from build123d import *

# Parameters (mm, degrees)
SKETCH9_R           = 25
BOSS_EXTRUDE7_DEPTH = 10


with BuildPart() as part:
    # Sketch9 → Boss-Extrude7 (new, symmetric)
    with BuildSketch(Plane(origin=(0, 0, 0), x_dir=(1, 0, 0), z_dir=(0, 1, 0))):
        with BuildLine():
            Line((0, -240), (140, -240))
            Line((140, -240), (43.894055239, 23.943932732))
            ThreePointArc((43.894055239, 23.943932732), (0, 50), (-43.894055239, 23.943932732))
            Line((-43.894055239, 23.943932732), (-140, -240))
            Line((-140, -240), (0, -240))
        make_face()
        with Locations(Location((0, 0, 0), (0, 0, 270))):
            Circle(SKETCH9_R, mode=Mode.SUBTRACT)
    extrude(amount=BOSS_EXTRUDE7_DEPTH, both=True)


solid = part.part
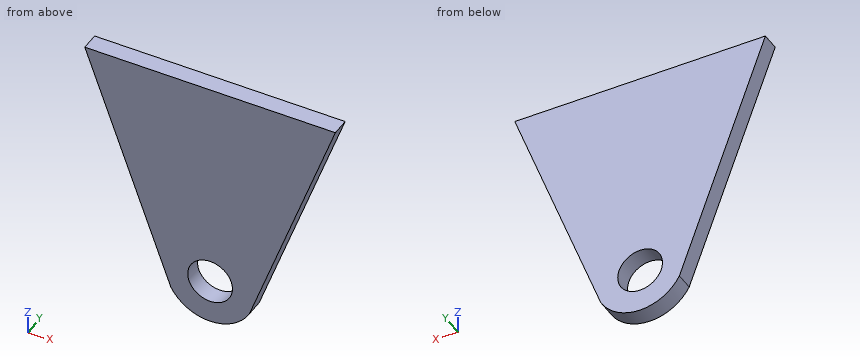
Design review of the part built by this model. Coordinates are the model's own, in mm. Round coordinates to 2 decimals unless told otherwise and drop trailing zeros. Write each loop counter-clockwise with the first axis right and the second up, starting at its lowest first coordinate (ties: lowest second). Pieces come first, ordered by that corner, then holes. Notation, with made-up numbers: (38, 76) - (81, 76) arc R21 cw to (81, 86) - close; hole circle Ø8 at (-18.75, 4). An arc over 180 degrees is marked (long way). Use a Markdown table: item, result. Add a question column.
1. We need section C-C (z = 0). State the section outline as (x, y) points, then the cut area to 3 significant figures.
2. Clearance check with flat-ended pins moving along their axes: pin 1 (6 mm diameter, centred on y = -4, z = 195.5, fed in from -X); pin 2 (12 mm diameter, centred on y = -1.5, z = 141.5, fed in from +X); pin 3 (6 mm diameter, centred on y = 7, z = 155, fed in from +X). State where each tip first meets the part, or that it passes through.
3. Wall thickness on probe 1 along X at (y, z) = (5.5, 0); probe 2 along X at (y, z) = (7.25, 20.5); probe 3 along Z at (x, y) = (-16, 3): over which ranges is each line inside the solid? List them lowest first.
4. We need section B-B (y = -2.25). State the section outline as (x, z) points, then the cut area to 3 significant figures.
5. We need section A-A (x = 0). State the section outline as (y, z) points.
6. We need section D-D (x = -74.5). State the section outline as (y, z) points.
Output:
| question | item | result |
|---|---|---|
| 1 | outline | (-52.61, -10) - (-25, -10) - (-25, 10) - (-52.61, 10) - close; (25, -10) - (52.61, -10) - (52.61, 10) - (25, 10) - close |
| 1 | area | 1,100 mm2 |
| 2 | pin 1 | stops at x = -124.89 |
| 2 | pin 2 | stops at x = 106.32 |
| 2 | pin 3 | stops at x = 110.14 |
| 3 | probe 1 | x = -52.61 to -25, 25 to 52.61 |
| 3 | probe 2 | x = -60.08 to -14.31, 14.31 to 60.08 |
| 3 | probe 3 | z = -47.37 to -19.21, 19.21 to 240 |
| 4 | outline | (-140, 240) - (-43.89, -23.94) arc R50 ccw to (43.89, -23.94) - (140, 240) - close; hole circle Ø50 at (0, 0) |
| 4 | area | 48,200 mm2 |
| 5 | outline | (-10, -50) - (10, -50) - (10, -25) - (-10, -25) - close; (-10, 25) - (10, 25) - (10, 240) - (-10, 240) - close |
| 6 | outline | (-10, 60.11) - (10, 60.11) - (10, 240) - (-10, 240) - close |
